Autodesk Inventor part; units mm, degrees
ref_plane "YZ Plane" through (0, 0, 0) normal (1, 0, 0) x (0, 1, 0)
ref_plane "XZ Plane" through (0, 0, 0) normal (0, 1, 0) x (-1, 0, 0)
ref_plane "XY Plane" through (0, 0, 0) normal (0, 0, 1) x (1, 0, 0)
sketch "Sketch1" plane through (0, 0, 0) normal (0, 0, 1) x (1, 0, 0)
  line L0 (0, 0) -> (-4, 0)
  line L1 (-4, 0) -> (-4, -4.15)
  line L2 (-4, -4.15) -> (0, -4.15)
  line L3 (0, -4.15) -> (0, 0)
  line L4 (0, 0) -> (-13.1356, 0) construction
  dimension "d1" = 4.15
  dimension "d2" = 4
revolve "Shoulder" add sketch "Sketch1" angle 360 about axis through (0, -4.15, 0) along (0, 1, 0)
sketch "Sketch2" plane through (0, 0, 0) normal (0, 1, 0) x (1, 0, 0)
  circle A0 centre (0, 0) radius 4
  circle A1 centre (0, 0) radius 3.76
  dimension "d3" = 7.52
extrude "Shoulder_neck" add sketch "Sketch2" along normal blind 1.85 contours A1
sketch "Sketch3" plane through (0, 1.85, 0) normal (0, 1, 0) x (1, 0, 0)
  circle A0 centre (0, 0) radius 3.76
  circle A1 centre (0, 0) radius 6.6
  dimension "d6" = 13.2
extrude "Head" add sketch "Sketch3" along normal blind 5.5 contours A0 | A1
sketch "Sketch4" plane through (0, -4.15, 0) normal (0, -1, 0) x (1, 0, 0)
  circle A0 centre (0, 0) radius 4
  circle A1 centre (0, 0) radius 2.255
  dimension "d9" = 4.51
extrude "Thread_neck" add sketch "Sketch4" along normal blind 2.3 contours A1
sketch "Sketch5" plane through (0, -6.45, 0) normal (0, -1, 0) x (1, 0, 0)
  circle A0 centre (0, 0) radius 2.255
  circle A1 centre (0, 0) radius 3
  dimension "d12" = 6
extrude "Thread_shoulder" add sketch "Sketch5" along normal blind 8.7 contours A0 | A1
sketch "Sketch6" plane through (0, 7.35, 0) normal (0, 1, 0) x (1, 0, 0)
  circle A0 centre (0, 0) radius 6.6
  circle A1 centre (0, 0) radius 2 construction
  line L0 (-2, 1.1547) -> (-2, -1.1547)
  line L1 (-2, -1.1547) -> (0, -2.3094)
  line L2 (0, -2.3094) -> (2, -1.1547)
  line L3 (2, -1.1547) -> (2, 1.1547)
  line L4 (2, 1.1547) -> (0, 2.3094)
  line L5 (0, 2.3094) -> (-2, 1.1547)
  dimension "d15" = 4
extrude "Hex" cut sketch "Sketch6" against normal blind 3.3 contours L5 L4 L3 L2 L1 L0
chamfer "Chamfer1" distance 0.24 angle 30 1 edges at (4, 0, 0) measured on face at (-3.8813, 0, -0.3191)
fillet "Fillet1" radius 0.4 1 edges at (-3.76, 1.85, 0)
chamfer "Chamfer2" distance 0.4 angle 30 1 edges at (-6.6, 7.35, 0) measured on face at (6.5145, 5.5167, 1.0587)
chamfer "Chamfer3" distance 0.5 angle 30 1 edges at (-3, -15.15, 0) measured on face at (-0.5351, -15.15, 1.0949)
fillet "Fillet2" radius 0.6 1 edges at (-2.255, -4.15, 0)
chamfer "Chamfer7" distance 0.745 angle 30 1 edges at (-3, -6.45, 0) measured on face at (2.7008, -6.45, -0.4192)
thread "Thread"
equation "\"d3\" = Shoulder_neck_dia"
equation "\"d4\" = Shoulder_neck_length"
equation "\"d6\" = Head_diameter"
equation "\"d7\" = Head_height"
equation "\"d9\" = Thread_neck_dia"
equation "\"d10\" = Thread_neck_length"
equation "\"d12\" = Thread_diameter"
equation "\"d13\" = Thread_length - Thread_neck_length"
equation "\"d15\" = Hex_size"
equation "\"d16\" = Hex_length"
equation "\"d18\" = -0.5 * Shoulder_neck_dia + 0.5 * Shoulder_diameter"
equation "\"d64\" = -0.5 * Shoulder_neck_dia + 0.5 * Shoulder_diameter"
equation "\"d21\" = 0.1 * Hex_size"
equation "\"d65\" = 0.1 * Hex_size"
equation "\"d23\" = 0.5 * Thread_pitch"
equation "\"d66\" = 0.5 * Thread_pitch"
equation "\"d25\" = Thread_neck_radius"
equation "\"d60\" = -0.5 * Thread_neck_dia + 0.5 * Thread_diameter"
equation "\"d67\" = -0.5 * Thread_neck_dia + 0.5 * Thread_diameter"
equation "\"d1\" = Shoulder_length - Shoulder_neck_length"
equation "\"d2\" = 0.5 * Shoulder_diameter"
equation "\"Shoulder_diameter\" = 8"
equation "\"Shoulder_length\" = 6"
equation "\"Shoulder_neck_dia\" = 7.52"
equation "\"Thread_diameter\" = 6"
equation "\"Thread_length\" = 11"
equation "\"Head_diameter\" = 13.2"
equation "\"Head_height\" = 5.5"
equation "\"Thread_neck_dia\" = 4.51"
equation "\"Hex_size\" = 4"
equation "\"Hex_length\" = 3.3"
equation "\"Thread_pitch\" = 1"
equation "\"Shoulder_neck_length\" = 1.85"
equation "\"Thread_neck_length\" = 2.3"
equation "\"Thread_neck_radius\" = 0.6"
properties part number "SCREW,SHOULDER,M8X6MM" material "Steel, High Strength Low Alloy"
Geometry check sheet. Reference: the model listing, model coordinates, mm. A direction names the side the tool comes from. Give positions to 0.01 mm unless a question says otherwise; leave off trailing zeros. Write each loop counter-clockwise with the first axis right and the second up, starting at its lowest first coordinate (ties: lowest second). Pieces come first, ordered by that corner, then holes. Notation, with made-up numbers: (-37.5, 14.5) - (19.5, 14.5) arc R8 ccw to (19.5, 21.5) - close; hole circle Ø8 at (-7, 14). An arc over 180 degrees is marked (long way). Put each result on its own line as item: value.
1. Draft check along X on faces 1 (the flat face through (-2, 6, 0)), 2 (the flat face through (0, -15.15, 0)), 3 (the cylindrical face through (2.083, -5.588, 0.864)). Enter one of: +X half, -X half, draft (parallel to the pull), parting line (faces both ways), or undercut.
Ans:
face 1: undercut
face 2: draft
face 3: parting line
2. Sectioned sample at A-A, the plane y = -8. Enter the section's corners in (x, z), plus the area to 3 significant figures.
Ans:
outline: circle Ø6 at (0, 0)
area: 28.3 mm²
3. Go/stop test with flat-tipped pins: pin 1 (3 mm diameter, centred on x = 4, y = -2.5, fed in from -Z); pin 2 (2 mm diameter, centred on y = 0, z = 3, fed in from -X); pin 3 (2 mm diameter, centred on x = 0, y = -4.5, fed in from +Z). Record where each tip stops, or that it passes through.
Ans:
pin 1: stops at z = -3.12
pin 2: stops at x = -3.46
pin 3: stops at z = 4
4. Thickness scan on line 1 (Y direction, x = 1, z = -5.25); line 2 (Y direction, x = -1.5, z = -0.25); line 3 (X direction, y = 6.5, z = 1). Record the ranges inside material, lowest first.
Ans:
line 1: y = 1.85 to 7.35
line 2: y = -15.15 to 4.05
line 3: x = -6.52 to -2, 2 to 6.52
5. Set-up check for faces 4 (the flat face through (1.014, 5.723, -1.724)), 5 (the cylindrical face through (-3, -11, 0)), 6 (the flat face through (-2, 7.35, -2)): record each of +Z, -Z, +X, -X, +Y, -Y from which the full face is reachable in a straight line by a thin tool's end or side.
Ans:
face 4: +Y
face 5: -Y
face 6: +Z, -Z, +X, -X, +Y
6. Sectioned sample at B-B, the plane y = -5. Enter the section's corners in (x, z) (3 decimals), plus the area to 3 significant figures.
Ans:
outline: circle Ø4.51 at (0, 0)
area: 16.0 mm²
